```python
from build123d import *

# Parameters (mm, degrees)
SKETCH1_R           = 2.5
BOSS_EXTRUDE1_DEPTH = 5


with BuildPart() as part:
    # Sketch1 → Boss-Extrude1 (new body)
    with BuildSketch(Plane(origin=(0, 0, 0), x_dir=(1, 0, 0), z_dir=(0, 1, 0))):
        Polygon((0, 0), (0, 230), (110, 230), (110, -35), (110, -40), (40, -40), align=None)
        with Locations((40, 220)):
            Circle(SKETCH1_R, mode=Mode.SUBTRACT)
        with Locations((100, 220)):
            Circle(SKETCH1_R, mode=Mode.SUBTRACT)
        with Locations((40, 185)):
            Circle(SKETCH1_R, mode=Mode.SUBTRACT)
        with Locations((100, 185)):
            Circle(SKETCH1_R, mode=Mode.SUBTRACT)
        with Locations((40, 150)):
            Circle(SKETCH1_R, mode=Mode.SUBTRACT)
        with Locations((100, 150)):
            Circle(SKETCH1_R, mode=Mode.SUBTRACT)
        with Locations((40, 115)):
            Circle(SKETCH1_R, mode=Mode.SUBTRACT)
        with Locations((100, 115)):
            Circle(SKETCH1_R, mode=Mode.SUBTRACT)
        with Locations((40, 80)):
            Circle(SKETCH1_R, mode=Mode.SUBTRACT)
        with Locations((100, 80)):
            Circle(SKETCH1_R, mode=Mode.SUBTRACT)
        with Locations((40, 45)):
            Circle(SKETCH1_R, mode=Mode.SUBTRACT)
        with Locations((100, 45)):
            Circle(SKETCH1_R, mode=Mode.SUBTRACT)
        with Locations((40, 10)):
            Circle(SKETCH1_R, mode=Mode.SUBTRACT)
        with Locations((100, 10)):
            Circle(SKETCH1_R, mode=Mode.SUBTRACT)
        with Locations((40, -25)):
            Circle(SKETCH1_R, mode=Mode.SUBTRACT)
        with Locations((100, -25)):
            Circle(SKETCH1_R, mode=Mode.SUBTRACT)
    extrude(amount=BOSS_EXTRUDE1_DEPTH)


solid = part.part
```
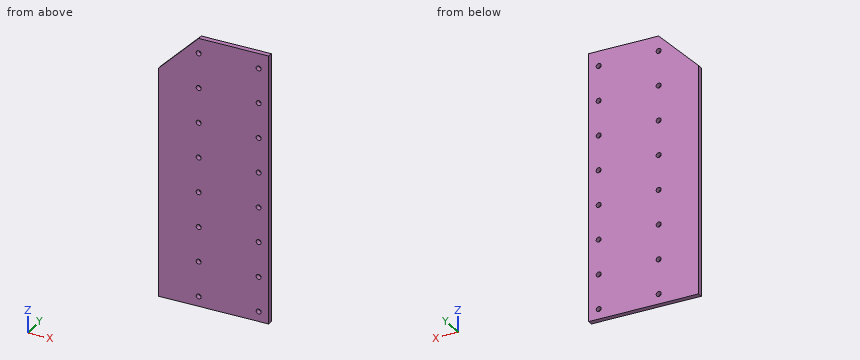
CAD build for the part. Positions are in the model's coordinates, mm. Give positions to 0.01 mm unless a question says otherwise; leave off trailing zeros. Write each loop counter-clockwise with the first axis right and the second up, starting at its lowest first coordinate (ties: lowest second). Pieces come first, ordered by that corner, then holes. Notation, with made-up numbers: (-1.75, -14.75) -> (47.25, -14.75) arc R8 cw to (47.25, -5.75) -> close; hole circle Ø4 at (23.5, -32.75). An arc over 180 degrees is marked (long way). Write each question's results on one line, items separated by ' | '.
1. Cut at B-B, the plane y = 3.7. Give the number of separate pieces and of enclosed holes in the cut face, then the cut area to 3 significant figures.
Geometry check:
separate pieces: 1 | enclosed holes: 16 | area: 28,600 mm²
2. Cut at A-A, the plane z = -80. Write the cut outline in (x, y).
Geometry check:
outline: (0, 0) -> (37.5, 0) -> (37.5, 5) -> (0, 5) -> close; (42.5, 0) -> (97.5, 0) -> (97.5, 5) -> (42.5, 5) -> close; (102.5, 0) -> (110, 0) -> (110, 5) -> (102.5, 5) -> close
3. Cut at D-D, the plane x = 22. Write the cut outline in (y, z).
Geometry check:
outline: (0, -230) -> (5, -230) -> (5, 22) -> (0, 22) -> close
4. Wall check: probe 1 along X at (y, z) = (3.3, -80); probe 2 along X at (y, z) = (3.8, 25); probe 3 along Z at (x, y) = (5.5, 2.1). Give the ranges that are in metal, low to high. Write a range as [from, to].
Geometry check:
probe 1: [0, 37.5], [42.5, 97.5], [102.5, 110] | probe 2: [25, 37.5], [42.5, 97.5], [102.5, 110] | probe 3: [-230, 5.5]
